```python
from build123d import *

# Parameters (mm, degrees)
BOSS_EXTRUDE1_DEPTH = 70
BOSS_EXTRUDE3_REACH = 86.63
SKETCH3_W           = 1.8
SKETCH3_H           = 3.8
SKETCH4_W           = 5
SKETCH4_H           = 3
BOSS_EXTRUDE4_DEPTH = 2
CUT_EXTRUDE1_REACH  = 90.595
SKETCH5_R           = 1.5
CUT_EXTRUDE2_REACH  = 86.63
SKETCH6_R           = 5


with BuildPart() as part:
    # Sketch1 → Boss-Extrude1 (new body)
    with BuildSketch(Plane.XY):
        with BuildLine():
            Line((-30.398230088, 19.964424779), (-30.398230088, -13.495575221))
            ThreePointArc((-30.398230088, -13.495575221), (-28.708236216, -17.575581349), (-24.628230088, -19.265575221))
            Line((-24.628230088, -19.265575221), (9.601769912, -19.265575221))
            Line((9.601769912, -19.265575221), (9.601769912, -17.265575221))
            Line((9.601769912, -17.265575221), (-24.628230088, -17.265575221))
            ThreePointArc((-24.628230088, -17.265575221), (-27.294022654, -16.161367786), (-28.398230088, -13.495575221))
            Line((-28.398230088, -13.495575221), (-28.398230088, 19.964424779))
            ThreePointArc((-28.398230088, 19.964424779), (-27.294022654, 22.630217344), (-24.628230088, 23.734424779))
            Line((-24.628230088, 23.734424779), (-10.398230088, 23.734424779))
            Line((-10.398230088, 23.734424779), (-10.398230088, 25.734424779))
            Line((-10.398230088, 25.734424779), (-24.628230088, 25.734424779))
            ThreePointArc((-24.628230088, 25.734424779), (-28.708236216, 24.044430906), (-30.398230088, 19.964424779))
        make_face()
    extrude(amount=BOSS_EXTRUDE1_DEPTH)

    # Sketch3 → Boss-Extrude3 (add, up to next)
    with BuildSketch(Plane(origin=(9.601769912, 0, 0), x_dir=(0, 0, -1), z_dir=(1, 0, 0)), mode=Mode.PRIVATE) as boss_extrude3_sk1:
        with Locations((-69.1, -15.365575221)):
            Rectangle(SKETCH3_W, SKETCH3_H)
    boss_extrude3_tool1 = extrude(boss_extrude3_sk1.sketch, amount=-BOSS_EXTRUDE3_REACH, mode=Mode.PRIVATE) - part.part
    # Sketch3 → Boss-Extrude3 (add, up to next)
    with BuildSketch(Plane(origin=(9.601769912, 0, 0), x_dir=(0, 0, -1), z_dir=(1, 0, 0)), mode=Mode.PRIVATE) as boss_extrude3_sk2:
        with Locations((-0.9, -15.365575221)):
            Rectangle(SKETCH3_W, SKETCH3_H)
    boss_extrude3_tool2 = extrude(boss_extrude3_sk2.sketch, amount=-BOSS_EXTRUDE3_REACH, mode=Mode.PRIVATE) - part.part
    add(boss_extrude3_tool1.solids().sort_by_distance((9.60177, -15.365575, 69.1))[0])
    add(boss_extrude3_tool2.solids().sort_by_distance((9.60177, -15.365575, 0.9))[0])

    # Sketch4 → Boss-Extrude4 (add)
    with BuildSketch(Plane(origin=(0, -13.465575221, 0), x_dir=(1, 0, 0), z_dir=(0, 1, 0))):
        with Locations((7.101769912, -68.5)):
            Rectangle(SKETCH4_W, SKETCH4_H)
        with Locations((7.101769912, -1.5)):
            Rectangle(SKETCH4_W, SKETCH4_H)
    extrude(amount=BOSS_EXTRUDE4_DEPTH)

    # Sketch5 → Cut-Extrude1 (cut, up to next)
    with BuildSketch(Plane(origin=(0, -19.265575221, 0), x_dir=(-1, 0, 0), z_dir=(0, -1, 0)), mode=Mode.PRIVATE) as cut_extrude1_sk1:
        with Locations(Location((17.128230088, -60, 0), (0, 0, 180))):
            Circle(SKETCH5_R)
    cut_extrude1_tool1 = extrude(cut_extrude1_sk1.sketch, amount=-CUT_EXTRUDE1_REACH, mode=Mode.PRIVATE) & part.part
    # Sketch5 → Cut-Extrude1 (cut, up to next)
    with BuildSketch(Plane(origin=(0, -19.265575221, 0), x_dir=(-1, 0, 0), z_dir=(0, -1, 0)), mode=Mode.PRIVATE) as cut_extrude1_sk2:
        with Locations(Location((17.128230088, -10, 0), (0, 0, 90))):
            Circle(SKETCH5_R)
    cut_extrude1_tool2 = extrude(cut_extrude1_sk2.sketch, amount=-CUT_EXTRUDE1_REACH, mode=Mode.PRIVATE) & part.part
    # Sketch5 → Cut-Extrude1 (cut, up to next)
    with BuildSketch(Plane(origin=(0, -19.265575221, 0), x_dir=(-1, 0, 0), z_dir=(0, -1, 0)), mode=Mode.PRIVATE) as cut_extrude1_sk3:
        with Locations(Location((-2.871769912, -51.67, 0), (0, 0, 180))):
            Circle(SKETCH5_R)
    cut_extrude1_tool3 = extrude(cut_extrude1_sk3.sketch, amount=-CUT_EXTRUDE1_REACH, mode=Mode.PRIVATE) & part.part
    # Sketch5 → Cut-Extrude1 (cut, up to next)
    with BuildSketch(Plane(origin=(0, -19.265575221, 0), x_dir=(-1, 0, 0), z_dir=(0, -1, 0)), mode=Mode.PRIVATE) as cut_extrude1_sk4:
        with Locations(Location((-2.871769912, -18.33, 0), (0, 0, 90))):
            Circle(SKETCH5_R)
    cut_extrude1_tool4 = extrude(cut_extrude1_sk4.sketch, amount=-CUT_EXTRUDE1_REACH, mode=Mode.PRIVATE) & part.part
    add(cut_extrude1_tool1.solids().sort_by_distance((-17.12823, -19.265575, 60))[0], mode=Mode.SUBTRACT)
    add(cut_extrude1_tool2.solids().sort_by_distance((-17.12823, -19.265575, 10))[0], mode=Mode.SUBTRACT)
    add(cut_extrude1_tool3.solids().sort_by_distance((2.87177, -19.265575, 51.67))[0], mode=Mode.SUBTRACT)
    add(cut_extrude1_tool4.solids().sort_by_distance((2.87177, -19.265575, 18.33))[0], mode=Mode.SUBTRACT)

    # Sketch6 → Cut-Extrude2 (cut, up to next)
    with BuildSketch(Plane.ZY.offset(30.398230088), mode=Mode.PRIVATE) as cut_extrude2_sk1:
        with Locations(Location((5.8, -9.065575221, 0), (0, 0, 297.625166054))):
            Circle(SKETCH6_R)
    cut_extrude2_tool1 = extrude(cut_extrude2_sk1.sketch, amount=-CUT_EXTRUDE2_REACH, mode=Mode.PRIVATE) & part.part
    add(cut_extrude2_tool1.solids().sort_by_distance((-30.39823, -9.065575, 5.8))[0], mode=Mode.SUBTRACT)


solid = part.part
```
The model under review builds one solid part; all positions refer to its coordinate system, in mm. A direction names the side the tool comes from. Round coordinates to 2 decimals unless told otherwise and drop trailing zeros. Loops run counter-clockwise (first coordinate to the right, second up) from the corner with the lowest first, then second, coordinate; pieces in that order, holes last. Notation, with made-up numbers: M -5,27 L 28,27 A13 cw 28,50 Z; hole C -13,-37.75 d7. An arc over 180 degrees is marked long. Answer as a JSON object with one key per item and string values.
(1) Clearance check with flat-ended pins moving along their axes: P1, Ø0.9, axis at x = 7.5, z = 68.5, coming from the +Y side; P2, Ø1, axis at y = 24.5, z = 26, coming from the +X side; P3, Ø1.8, axis at x = 2.87, z = 18.33, coming from the +Y side; P4, Ø3, axis at x = -26.5, z = 31, coming from the -Y side. State where each tip first meets the part, or that it passes through.
Resolved:
{"P1": "y = -11.47", "P2": "x = -10.4", "P3": "through", "P4": "y = -19.25"}
(2) Take a section at D-D on z = 60. Give the boundary of the cut face in (x, y).
Resolved:
{"outline": "M -30.4,-13.5 A5.77 ccw -24.63,-19.27 L -18.63,-19.27 L -18.63,-17.27 L -24.63,-17.27 A3.77 cw -28.4,-13.5 L -28.4,19.96 A3.77 cw -24.63,23.73 L -10.4,23.73 L -10.4,25.73 L -24.63,25.73 A5.77 ccw -30.4,19.96 Z; M -15.63,-19.27 L 9.6,-19.27 L 9.6,-17.27 L -15.63,-17.27 Z"}
(3) Take a section at B-B on x = -23. Give the boundary of the cut face in (y, z), and give its area (3 significant figures).
Resolved:
{"outline": "M -19.27,0 L -13.47,0 L -13.47,1.8 L -17.27,1.8 L -17.27,68.2 L -13.47,68.2 L -13.47,70 L -19.27,70 Z; M 23.73,0 L 25.73,0 L 25.73,70 L 23.73,70 Z", "area": "294 mm²"}
(4) Tool access review of faces 4 (the flat face through (-12, -13.466, 1)), 5 (the flat face through (7, -11.466, 68)), 6 (the cylindrical face through (-27.265, -16.191, 34.535)): name each direction out of +Z, -Z, +X, -X, +Y, -Y from which nothing blocks a thin tool from reaching the whole face with its end or side.
Resolved:
{"face 4": "+Z, -Z", "face 5": "+Z, -Z, +X, +Y", "face 6": "+X"}
(5) Take a section at A-A on z = 5.8. Give the boundary of the cut face in (x, y).
Resolved:
{"outline": "M -30.4,-4.07 L -28.4,-4.07 L -28.4,19.96 A3.77 cw -24.63,23.73 L -10.4,23.73 L -10.4,25.73 L -24.63,25.73 A5.77 ccw -30.4,19.96 Z; M -30.37,-14.07 A5.77 ccw -24.63,-19.27 L 9.6,-19.27 L 9.6,-17.27 L -24.63,-17.27 A3.77 cw -28.35,-14.07 Z"}
(6) To check wall thickness, follow line 1 along Y through (x, z) = (-15, 13); line 2 along Y through (x, z) = (1.5, 29); line 3 along X through (y, z) = (-11.5, 47.5). State the ranges of each line that lie inside material, in increasing order.
Resolved:
{"line 1": "-19.27 to -17.27, 23.73 to 25.73", "line 2": "-19.27 to -17.27", "line 3": "-30.4 to -28.4"}
(7) Draft analysis for pull direction X (two halves, no side actions). For faces 1 (the flat face through (4.602, -12, 2)), 2 (the flat face through (-30.398, 3, 35)), 3 (the flat face through (-8, -19.266, 35)), state which applies: released by +X, released by -X, zero draft, split by the parting line, or undercut.
Resolved:
{"face 1": "undercut", "face 2": "released by -X", "face 3": "zero draft"}
(8) Take a section at C-C on z = 42.5. Give the boundary of the cut face in (x, y).
Resolved:
{"outline": "M -30.4,-13.5 A5.77 ccw -24.63,-19.27 L 9.6,-19.27 L 9.6,-17.27 L -24.63,-17.27 A3.77 cw -28.4,-13.5 L -28.4,19.96 A3.77 cw -24.63,23.73 L -10.4,23.73 L -10.4,25.73 L -24.63,25.73 A5.77 ccw -30.4,19.96 Z"}
